Autodesk Inventor part; units mm, degrees
ref_plane "YZ Plane" through (0, 0, 0) normal (1, 0, 0) x (0, 1, 0)
ref_plane "XZ Plane" through (0, 0, 0) normal (0, 1, 0) x (-1, 0, 0)
ref_plane "XY Plane" through (0, 0, 0) normal (0, 0, 1) x (1, 0, 0)
sketch "Sketch1" plane through (0, 0, 0) normal (0, 1, 0) x (-1, 0, 0)
  line L0 (0, 0) -> (150, 0)
  line L1 (150, 0) -> (150, -50)
  line L2 (150, -50) -> (0, -50)
  line L3 (0, -50) -> (0, 0)
  dimension "d0" = 150
  dimension "d1" = 50
extrude "Extrusion1" add sketch "Sketch1" along normal blind 10
sketch "Sketch2" plane through (0, 10, 0) normal (0, 1, 0) x (1, 0, 0)
  line L0 (-150, 50) -> (-150, 0)
  line L1 (-150, 0) -> (-138.3436, 0)
  line L2 (-138.3436, 0) -> (-138.3436, 50)
  line L3 (-138.3436, 50) -> (-150, 50)
  line L4 (-150, 50) -> (-150, 0)
  point P0 (0, 0)
extrude "Extrusion2" add sketch "Sketch2" along normal blind 90
fillet "Fillet1" radius 15 1 edges at (-138.3436, 10, -25)
fillet "Fillet2" radius 7.5 2 edges at (-138.3436, 100, -25) (0, 10, -25)
sketch "Sketch3" plane through (-138.3436, 25, 0) normal (1, 0, 0) x (0, 0, -1)
  line L0 (0, 0) -> (0, 67.5)
  line L1 (50, 0) -> (50, 67.5)
  line L2 (0, 67.5) -> (50, 67.5)
  line L3 (0, 0) -> (0, 67.5)
  line L4 (50, 0) -> (0, 0)
  line L5 (50, 0) -> (50, 67.5)
  circle A0 centre (25, 54) radius 4
  circle A1 centre (25, 13.5) radius 4
  point P0 (0, -25)
  dimension "d8" = 8
  dimension "d9" = 8
  dimension "d10" = 67.5
  dimension "d11" = 50
  dimension "d12" = 25
  dimension "d13" = 13.5
  dimension "d14" = 13.5
  dimension "d17" = 40.5
extrude "Extrusion3" cut sketch "Sketch3" against normal up to next contours A0 | A1
sketch "Sketch4" plane through (0, 0, 0) normal (0, -1, 0) x (1, 0, 0)
  line L0 (-150, 0) -> (-150, -50)
  circle A0 centre (-50, -25) radius 4.25
  line L1 (0, 0) -> (-150, 0)
  dimension "d18" = 8.5
  dimension "d19" = 100
  dimension "d20" = 50
  dimension "d21" = 25
extrude "Extrusion4" cut sketch "Sketch4" against normal blind 10
equation "\"d12\" = 0.5 * d11"
equation "\"d13\" = 0.2 * d10"
equation "\"d14\" = d13"
equation "\"d21\" = 0.5 * d20"
properties part number "L_ShapedBracket_100x200x10_ozce"
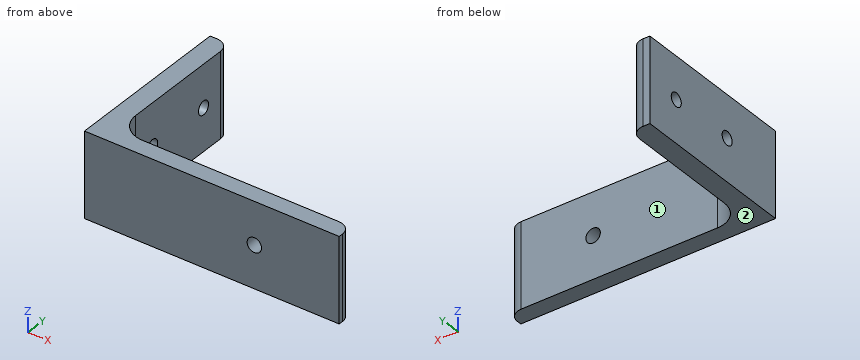
Could you check a few things on this model? Use its own coordinates, in mm. Face numbers are marked on the shaded views. A direction names the side the tool comes from. Coordinates: 2 decimals unless noted, no trailing zeros. Write each loop counter-clockwise with the first axis right and the second up, starting at its lowest first coordinate (ties: lowest second). Pieces come first, ordered by that corner, then holes. Notation, with made-up numbers: (51, -19.75) -> (56, -19.75) arc R21 cw to (56, -7.75) -> close; hole circle Ø5 at (-8, -12.75). An arc over 180 degrees is marked (long way). Return JSON: item names as keys, results as strings.
(1) I need wall thicknesses on L1, parallel to Z at x = -50, y = 3.5; L2, parallel to Y at x = -144, z = -25; L3, parallel to X at y = 55.5, z = -13. Which ranges of each line are inside material? Lowest first, please.
Numbers:
{"L1": "z = -50 to -29.25, -20.75 to 0", "L2": "y = 0 to 34.5, 42.5 to 75, 83 to 99.77", "L3": "x = -150 to -138.34"}
(2) I'm going to push flat-ended pins straight in: pin 1 (1.5 mm diameter, centred on y = 20.5, z = -41.5, fed in from +X); pin 2 (6.5 mm diameter, centred on y = 38.5, z = -25, fed in from +X); pin 3 (10 mm diameter, centred on x = -29, z = -36, fed in from +Y); pin 4 (10 mm diameter, centred on y = 24.5, z = -34.5, fed in from +X). Where does each tip first touch, or does it pass through?
Numbers:
{"pin 1": "stops at x = -137.39", "pin 2": "passes through", "pin 3": "stops at y = 10", "pin 4": "stops at x = -137.3"}
(3) Imagine slicing it at A-A, the plane z = -25. Please give me the cut outline in (x, y).
Numbers:
{"outline": "(-150, 0) -> (-54.25, 0) -> (-54.25, 10) -> (-123.34, 10) arc R15 cw to (-138.34, 25) -> (-138.34, 34.5) -> (-150, 34.5) -> close; (-150, 42.5) -> (-138.34, 42.5) -> (-138.34, 75) -> (-150, 75) -> close; (-150, 83) -> (-138.34, 83) -> (-138.34, 92.5) arc R7.5 ccw to (-145.84, 100) -> (-150, 100) -> close; (-45.75, 0) -> (0, 0) -> (0, 2.5) arc R7.5 ccw to (-7.5, 10) -> (-45.75, 10) -> close"}
(4) Imagine slicing it at C-C, the plane x = -50. Please give me the cut outline in (y, z).
Numbers:
{"outline": "(0, -50) -> (10, -50) -> (10, -29.25) -> (0, -29.25) -> close; (0, -20.75) -> (10, -20.75) -> (10, 0) -> (0, 0) -> close"}
(5) Imagine slicing it at B-B, the plane y = 79. Please give me the cut outline in (x, z), then the cut area to 3 significant figures.
Numbers:
{"outline": "(-150, -50) -> (-138.34, -50) -> (-138.34, -29) -> (-150, -29) -> close; (-150, -21) -> (-138.34, -21) -> (-138.34, 0) -> (-150, 0) -> close", "area": "490 mm2"}
(6) Imagine slicing it at D-D, the plane z = -5.5. Please give me the cut outline in (x, y).
Numbers:
{"outline": "(-150, 0) -> (0, 0) -> (0, 2.5) arc R7.5 ccw to (-7.5, 10) -> (-123.34, 10) arc R15 cw to (-138.34, 25) -> (-138.34, 92.5) arc R7.5 ccw to (-145.84, 100) -> (-150, 100) -> close"}
(7) Which directions (+Z, -Z, +X, -X, +Y, -Y) give clear straight access to the entire face, cutting with the end or side of a thin tool? Please do the marked faces 1 and 2.
Numbers:
{"face 1": "+Z, -Z, +X, +Y", "face 2": "-Z, +X, -X, +Y, -Y"}
